The listing builds one solid part. Answer for the finished solid, in the listing's coordinates (mm). Coordinates: 2 decimals unless noted, no trailing zeros. Order: outer loops, then holes, each group sorted by start corner. A loop starts at its lowest first (then second) coordinate and runs counter-clockwise, first axis right, second up. Notation, with made-up numbers: (-28.75, 55.5) -> (1.25, 55.5) arc R27 cw to (1.25, 89.5) -> close; hole circle Ø8 at (80.25, 63). An arc over 180 degrees is marked (long way). Write item = value, one per line.
from build123d import *

# Parameters (mm, degrees)
F0_W     = 19.5166560506
F0_H     = 12.7
F0_W_2   = 16.3915466189
F0_H_2   = 13.060019505
F1_DEPTH = 5.08
F0_H_3   = 2.5634752994
F2_DEPTH = 5.08
F3_DEPTH = 3.81
F4_DEPTH = 3.81


with BuildPart() as f1:
    # F0 (on Top) → F1 (new body)
    with BuildSketch(Plane.XY):
        Polygon((-86.9376676773, 107.6591225748), (-86.9376676773, 120.3591225748), (-145.258925468, 120.3591225748), (-145.258925468, -120.9408774252), (90.1978743578, -120.9408774252), (90.1978743578, -107.8808579201), (-126.208925468, -107.8808579201), (-126.208925468, -44.3808579201), (-126.208925468, 107.6591225748), align=None)
        Polygon((146.841074532, -120.9408774252), (146.841074532, 120.3591225748), (-67.4210116267, 120.3591225748), (-67.4210116267, 107.6591225748), (127.791074532, 107.6591225748), (127.791074532, -107.8808579201), (106.5894209767, -107.8808579201), (106.5894209767, -120.9408774252), align=None)
        with Locations((-77.179339652, 114.0091225748)):
            Rectangle(F0_W, F0_H)
        with Locations((98.3936476673, -114.4108676727)):
            Rectangle(F0_W_2, F0_H_2)
    extrude(amount=F1_DEPTH)

    # F0 (on Top) → F2 (join)
    with BuildSketch(Plane.XY):
        Polygon((127.791074532, 107.6591225748), (-67.4210116267, 107.6591225748), (-67.4210116267, 105.0956472754), (-86.9376676773, 105.0956472754), (-86.9376676773, 107.6591225748), (-126.208925468, 107.6591225748), (-126.208925468, -44.3808579201), (-126.208925468, -107.8808579201), (90.1978743578, -107.8808579201), (106.5894209767, -107.8808579201), (127.791074532, -107.8808579201), align=None)
        with Locations((-77.179339652, 106.3773849251)):
            Rectangle(F0_W, F0_H_3)
    extrude(amount=F2_DEPTH)

    # F0 (on Top) → F3 (cut)
    with BuildSketch(Plane.XY):
        Polygon((127.791074532, 107.6591225748), (-67.4210116267, 107.6591225748), (-67.4210116267, 105.0956472754), (-86.9376676773, 105.0956472754), (-86.9376676773, 107.6591225748), (-126.208925468, 107.6591225748), (-126.208925468, -44.3808579201), (-126.208925468, -107.8808579201), (90.1978743578, -107.8808579201), (106.5894209767, -107.8808579201), (127.791074532, -107.8808579201), align=None)
        with Locations((-77.179339652, 106.3773849251)):
            Rectangle(F0_W, F0_H_3)
    extrude(amount=F3_DEPTH, mode=Mode.SUBTRACT)

    # F0 (on Top) → F4 (cut)
    with BuildSketch(Plane.XY):
        with Locations((98.3936476673, -114.4108676727)):
            Rectangle(F0_W_2, F0_H_2)
        with Locations((-77.179339652, 114.0091225748)):
            Rectangle(F0_W, F0_H)
    extrude(amount=F4_DEPTH, mode=Mode.SUBTRACT)


solid = f1.part
Q1. Section A-A, the plane z = 2.35 is taken. Give the vertices of the cut face in (x, y).
The answers:
outline = (-145.26, -120.94) -> (90.2, -120.94) -> (90.2, -107.88) -> (-126.21, -107.88) -> (-126.21, 107.66) -> (-86.94, 107.66) -> (-86.94, 120.36) -> (-145.26, 120.36) -> close; (-67.42, 107.66) -> (127.79, 107.66) -> (127.79, -107.88) -> (106.59, -107.88) -> (106.59, -120.94) -> (146.84, -120.94) -> (146.84, 120.36) -> (-67.42, 120.36) -> close
Q2. Section B-B, the plane y = 78.5 is taken. Give the vertices of the cut face in (x, z), plus the area to 3 significant figures.
The answers:
outline = (-145.26, 0) -> (-126.21, 0) -> (-126.21, 3.81) -> (127.79, 3.81) -> (127.79, 0) -> (146.84, 0) -> (146.84, 5.08) -> (-145.26, 5.08) -> close
area = 516 mm2
Q3. Section C-C, the plane x = -90 is taken. Give the vertices of the cut face in (y, z).
The answers:
outline = (-120.94, 0) -> (-107.88, 0) -> (-107.88, 3.81) -> (107.66, 3.81) -> (107.66, 0) -> (120.36, 0) -> (120.36, 5.08) -> (-120.94, 5.08) -> close
Q4. Find the intervals of material crossed by line 1 along X through (y, z) = (5, 1.3); line 2 along Y through (x, z) = (80.5, 2.6); line 3 along Z through (x, y) = (11, -60.5), in increasing order.
The answers:
line_1 = -145.26 to -126.21, 127.79 to 146.84
line_2 = -120.94 to -107.88, 107.66 to 120.36
line_3 = 3.81 to 5.08
Q5. The mould has two halves that part along Y. Classify faces 1 (the face through (-133, -27, 0)), 2 (the face through (-1, 1, 3.81)): released by +Y, released by -Y, zero draft, split by the parting line, or undercut.
The answers:
face_1 = zero draft
face_2 = undercut
Q6. This flat-tipped pin is pushed along its axis until it touches: pin 1 Ø12 at (x, y) = (-15, -20) entering from -Z. Where does it stop, or does it pass through?
The answers:
pin_1 = 3.81
